Autodesk Inventor part; units mm, degrees
ref_plane "YZ Plane" through (0, 0, 0) normal (1, 0, 0) x (0, 1, 0)
ref_plane "XZ Plane" through (0, 0, 0) normal (0, 1, 0) x (-1, 0, 0)
ref_plane "XY Plane" through (0, 0, 0) normal (0, 0, 1) x (1, 0, 0)
sketch "スケッチ1" plane through (0, 0, 0) normal (1, 0, 0) x (0, 1, 0)
  line L0 (-10, 5) -> (10, 5)
  line L1 (10, 5) -> (10, -5)
  line L2 (10, -5) -> (-10, -5)
  line L3 (-10, -5) -> (-10, 5)
  point P0 (0, 0)
  dimension "d0" = 20
  dimension "d2" = 10
  dimension "d3" = 10
  dimension "d4" = 5
extrude "押し出し1" add sketch "スケッチ1" along normal blind 4
sketch "スケッチ2" plane through (4, 0, 0) normal (1, 0, 0) x (0, 0, -1)
  line L0 (5, -10) -> (5, 10)
  line L1 (5, 10) -> (-5, 10)
  circle A0 centre (0, 5) radius 1
  circle A1 centre (0, -5) radius 1
  point P0 (0, 0)
  dimension "d7" = 2
  dimension "d9" = 10
  dimension "d10" = 5
  dimension "d11" = 5
  dimension "d12" = 5
hole "穴1" at (4, 5, 0) at (4, -5, 0) direction (-1, 0, 0) diameter 2 end through all
properties part number "Leg_Link_Shim" material "アセタール樹脂、白"
Part model, mm, in its own coordinate system. Coordinates: 2 decimals unless noted, no trailing zeros. Order: outer loops, then holes, each group sorted by start corner. A loop starts at its lowest first (then second) coordinate and runs counter-clockwise, first axis right, second up. Notation, with made-up numbers: (19.25, -20.5) - (44.25, -20.5) arc R16 ccw to (44.25, 3.5) - close; hole circle Ø11 at (-13, 68). An arc over 180 degrees is marked (long way). Use CSV: the item, a comma, the result in double quotes.
Item 1: Probe probe 1 along Y at (x, z) = (1.1, 0); probe 2 along Z at (x, y) = (1.55, 5); probe 3 along Z at (x, y) = (1.55, -5.5). List the from-to ranges inside material, lowest first.
Solved:
probe 1,"y = -10 to -6, -4 to 4, 6 to 10"
probe 2,"z = -5 to -1, 1 to 5"
probe 3,"z = -5 to -0.87, 0.87 to 5"
Item 2: Drop a flat-ended pin along its axis: P1, Ø2.5, axis at y = -5, z = 0, coming from the -X side. Give the stop position or say it passes through.
Solved:
P1,"stops at x = 0"
Item 3: Saw through at A-A on z = 0. Give the cut face in (x, y), and give its area (3 significant figures).
Solved:
outline,"(0, -10) - (4, -10) - (4, -6) - (0, -6) - close; (0, -4) - (4, -4) - (4, 4) - (0, 4) - close; (0, 6) - (4, 6) - (4, 10) - (0, 10) - close"
area,"64.0 mm²"
Item 4: Saw through at B-B on y = -5. Give the cut face in (x, z).
Solved:
outline,"(0, -5) - (4, -5) - (4, -1) - (0, -1) - close; (0, 1) - (4, 1) - (4, 5) - (0, 5) - close"
Item 5: Mould opens along Z. For faces 1 (the face through (2, 0, 5)), 2 (the face through (0, 0, 0)), 3 (the face through (2, 4, 0)) say: +Z half, -Z half, draft (parallel to the pull), parting line (faces both ways), or undercut.
Solved:
face 1,"+Z half"
face 2,"draft"
face 3,"undercut"
Item 6: Saw through at C-C on x = 1.6. Give the cut face in (y, z), and give its area (3 significant figures).
Solved:
outline,"(-10, -5) - (10, -5) - (10, 5) - (-10, 5) - close; hole circle Ø2 at (-5, 0); hole circle Ø2 at (5, 0)"
area,"194 mm²"
